from build123d import *

# Parameters (mm, degrees)
SKETCH5_W                    = 475.54896
SKETCH5_H                    = 260.35
BASE_FLANGE1_DEPTH           = 3.175
EDGE_FLANGE1_DEPTH           = 366.48136
EDGE_FLANGE2_STRIP_W         = 19.05
EDGE_FLANGE2_STRIP_H         = 3.175
EDGE_FLANGE2_STRIP_CUT_DEPTH = 260.35
EDGE_FLANGE2_DEPTH           = 260.35
EDGE_FLANGE3_DEPTH           = 260.35
CUT_EXTRUDE1_DEPTH           = 279.969149723
CUT_EXTRUDE1_DEPTH_BACK      = 279.969149723
SKETCH15_W                   = 329.647515686
SKETCH15_H                   = 175.541944057
CUT_EXTRUDE2_DEPTH           = 279.698003441
CUT_EXTRUDE2_DEPTH_BACK      = 279.698003441
SKETCH16_R                   = 12.065
SKETCH16_R_2                 = 1.524


# Sheet-metal steps are written as plain solids
with BuildPart() as part:
    # Sketch5 → Base-Flange1 (new body)
    with BuildSketch(Plane(origin=(0, 0, 0), x_dir=(1, 0, 0), z_dir=(0, 1, 0))):
        Rectangle(SKETCH5_W, SKETCH5_H)
    extrude(amount=-BASE_FLANGE1_DEPTH)

    # Edge-Flange1 section (across the edge) → Edge-Flange1 (add)
    with BuildSketch(Plane(origin=(128.70688, -3.175, 133.35), x_dir=(0, 0, -1), z_dir=(-1, 0, 0))):
        with BuildLine():
            Line((-3.175, 3.175), (-3.175, 15.875))
            Line((-3.175, 15.875), (0, 15.875))
            Line((0, 15.875), (0, 3.175))
            ThreePointArc((0, 3.175), (0.92993597, 0.92993597), (3.175, 0))
            Line((3.175, 0), (3.175, -3.175))
            ThreePointArc((3.175, -3.175), (-1.315128061, -1.315128061), (-3.175, 3.175))
        make_face()
    extrude(amount=EDGE_FLANGE1_DEPTH)

    # Edge-Flange2 strip (across the edge) → Edge-Flange2 strip cut (cut)
    with BuildSketch(Plane(origin=(237.77448, -3.175, -130.175), x_dir=(-1, 0, 0), z_dir=(0, 0, 1))):
        with Locations((-3.175, -1.5875)):
            Rectangle(EDGE_FLANGE2_STRIP_W, EDGE_FLANGE2_STRIP_H)
    extrude(amount=EDGE_FLANGE2_STRIP_CUT_DEPTH, mode=Mode.SUBTRACT)

    # Edge-Flange2 section (across the edge) → Edge-Flange2 (add)
    with BuildSketch(Plane(origin=(237.77448, -3.175, -130.175), x_dir=(-1, 0, 0), z_dir=(0, 0, 1))):
        with BuildLine():
            Line((0, 3.175), (0, 22.225))
            Line((0, 22.225), (3.175, 22.225))
            Line((3.175, 22.225), (3.175, 3.175))
            ThreePointArc((3.175, 3.175), (4.10493597, 0.92993597), (6.35, 0))
            Line((6.35, 0), (6.35, -3.175))
            ThreePointArc((6.35, -3.175), (1.859871939, -1.315128061), (0, 3.175))
        make_face()
    extrude(amount=EDGE_FLANGE2_DEPTH)

    # Edge-Flange3 section (across the edge) → Edge-Flange3 (add)
    with BuildSketch(Plane(origin=(-238.77448, -3.175, 130.175), x_dir=(1, 0, 0), z_dir=(0, 0, -1))):
        with BuildLine():
            Line((-3.175, 1), (-3.175, 22.225))
            Line((-3.175, 22.225), (0, 22.225))
            Line((0, 22.225), (0, 1))
            ThreePointArc((0, 1), (0.292893219, 0.292893219), (1, 0))
            Line((1, 0), (1, -3.175))
            ThreePointArc((1, -3.175), (-1.952170811, -1.952170811), (-3.175, 1))
        make_face()
    extrude(amount=EDGE_FLANGE3_DEPTH)

    # Sketch15 → Cut-Extrude1 (cut, two sides: drawn at the far end of the back side and taken through both)
    with BuildSketch(Plane(origin=(0, 0, 0), x_dir=(1, 0, 0), z_dir=(0, 1, 0)).offset(-CUT_EXTRUDE1_DEPTH_BACK)):
        with Locations((164.823757843, 154.445972028)):
            Rectangle(SKETCH15_W, SKETCH15_H)
    extrude(amount=CUT_EXTRUDE1_DEPTH + CUT_EXTRUDE1_DEPTH_BACK, mode=Mode.SUBTRACT)

    # Sketch16 → Cut-Extrude2 (cut, two sides: drawn at the far end of the back side and taken through both)
    with BuildSketch(Plane.XZ.offset(3.175).offset(-CUT_EXTRUDE2_DEPTH_BACK)):
        with Locations(Location((-191.14948, -92.075, 0), (0, 0, 270))):
            Circle(SKETCH16_R)
        with Locations(Location((-179.654811625, -80.580212705, 0), (0, 0, 270))):
            Circle(SKETCH16_R_2)
        with Locations(Location((-202.644148375, -80.580212705, 0), (0, 0, 270))):
            Circle(SKETCH16_R_2)
        with Locations(Location((-179.654811625, -103.569787295, 0), (0, 0, 90))):
            Circle(SKETCH16_R_2)
        with Locations(Location((-202.644148375, -103.569787295, 0), (0, 0, 90))):
            Circle(SKETCH16_R_2)
        with Locations(Location((-165.814148375, -80.580212705, 0), (0, 0, 270))):
            Circle(SKETCH16_R_2)
        with Locations(Location((-154.31948, -92.075, 0), (0, 0, 270))):
            Circle(SKETCH16_R)
        with Locations(Location((-142.824811625, -80.580212705, 0), (0, 0, 270))):
            Circle(SKETCH16_R_2)
        with Locations(Location((-165.814148375, -103.569787295, 0), (0, 0, 90))):
            Circle(SKETCH16_R_2)
        with Locations(Location((-142.824811625, -103.569787295, 0), (0, 0, 90))):
            Circle(SKETCH16_R_2)
    extrude(amount=CUT_EXTRUDE2_DEPTH + CUT_EXTRUDE2_DEPTH_BACK, mode=Mode.SUBTRACT)


solid = part.part
Source: CAD feature listing. Evaluate the final solid. Frame: model axes, mm. A direction names the side the tool comes from. Give positions to 0.01 mm unless a question says otherwise; leave off trailing zeros. Write each loop counter-clockwise with the first axis right and the second up, starting at its lowest first coordinate (ties: lowest second). Pieces come first, ordered by that corner, then holes. Notation, with made-up numbers: (-11.75, 75.25) -> (30.25, 75.25) arc R33 ccw to (30.25, 114.25) -> close; hole circle Ø11 at (75.25, 67.5). An arc over 180 degrees is marked (long way). Write item = value, one per line.
Q1. Cut plane C-C on z = -20.5. Return loops of the section in (x, y) (3 decimals), then the cut area to 3 significant figures.
Here are the results:
outline = (-241.949, -25.4) -> (-238.774, -25.4) -> (-238.774, -4.175) arc R1 cw to (-237.774, -3.175) -> (231.424, -3.175) arc R3.175 cw to (234.599, -6.35) -> (234.599, -25.4) -> (237.774, -25.4) -> (237.774, -6.35) arc R6.35 ccw to (231.424, 0) -> (-237.774, 0) arc R4.175 ccw to (-241.949, -4.175) -> close
area = 1,650 mm²
Q2. Cut plane A-A on y = -14.75. Return loops of the section in (x, z) (3 decimals).
Here are the results:
outline = (-241.949, -130.175) -> (-238.774, -130.175) -> (-238.774, 130.175) -> (-241.949, 130.175) -> close; (-237.774, 133.35) -> (128.707, 133.35) -> (128.707, 136.525) -> (-237.774, 136.525) -> close; (234.599, -66.675) -> (237.774, -66.675) -> (237.774, 130.175) -> (234.599, 130.175) -> close
Q3. Reachability of faces 1 (the face through (-52, -13, 133.35)), 2 (the face through (-6, -3.175, -2)), 3 (the face through (-238.774, -15, 2)) from +Z, -Z, +X, -X, +Y, -Y: full face, straight path, thin tool, end or side. Return the list, or none.
Here are the results:
face_1 = -Z, +X, -X, -Y
face_2 = -Z, -Y
face_3 = +Z, -Z, -Y
Q4. Line query: line 1 (X direction, y = -15.75, z = 21); line 2 (Y direction, x = -52.5, z = -79) (3 decimals); line 3 (Z direction, x = -42.5, y = -7) (3 decimals). Output: solid intervals per line, ascending. Write a range as from..to.
Here are the results:
line_1 = -241.95..-238.77, 234.6..237.77
line_2 = -3.175..0
line_3 = 133.35..136.525
Q5. Cut plane D-D on x = 4.5. Return loops of the section in (y, z) (3 decimals), then the cut area to 3 significant figures.
Here are the results:
outline = (-19.05, 133.35) -> (-6.35, 133.35) arc R3.175 cw to (-3.175, 130.175) -> (-3.175, -66.675) -> (0, -66.675) -> (0, 130.175) arc R6.35 ccw to (-6.35, 136.525) -> (-19.05, 136.525) -> close
area = 689 mm²
Q6. Cut plane B-B on x = -120. Return loops of the section in (y, z) (3 decimals).
Here are the results:
outline = (-19.05, 133.35) -> (-6.35, 133.35) arc R3.175 cw to (-3.175, 130.175) -> (-3.175, -130.175) -> (0, -130.175) -> (0, 130.175) arc R6.35 ccw to (-6.35, 136.525) -> (-19.05, 136.525) -> close
Q7. First-contact query: pin 1 (3.5 mm diameter, centred on x = -179.65, z = -80.58, fed in from -Y) (3 decimals); pin 2 (1.3 mm diameter, centred on x = -240, y = -15, fed in from +Z) (3 decimals); pin 3 (10 mm diameter, centred on x = -92.5, y = -12.5, fed in from -Z). Flat tips, straight axial feed; report the tip coordinate or a pass-through.
Here are the results:
pin_1 = -3.175
pin_2 = 130.175
pin_3 = 133.35
Q8. Mould query, pull axis X, two halves, no side actions, for faces 4 (the face through (118, -1, -66.675)), 5 (the face through (237.774, -16, 30)), 6 (the face through (-202.928, -1.565, -89.46)), 7 (the face through (-241.949, -15, 2)). Classes: +X half, -X half, draft (parallel to the pull), parting line (faces both ways), or undercut.
Here are the results:
face_4 = draft
face_5 = +X half
face_6 = undercut
face_7 = -X half
